Read the model definition and answer for the solid it produces. Units are mm, in the model's axes. Face numbers are marked on the shaded views. Give positions to 0.01 mm unless a question says otherwise; leave off trailing zeros. Write each loop counter-clockwise with the first axis right and the second up, starting at its lowest first coordinate (ties: lowest second). Pieces come first, ordered by that corner, then holes. Notation, with made-up numbers: (50.5, 19.5) -> (78.5, 19.5) arc R33 ccw to (78.5, 57.5) -> close; hole circle Ø5 at (71, -33). An arc over 180 degrees is marked (long way). Answer as CSV lines item,"result". Start each with the question number.
1. The part is cut by section A-A, the plane y = 0. Determine the outline of the cut face in (x, z) (3 decimals), and give its area (4 significant figures).
2. Given pin 1 (1 mm diameter, centred on x = 1.5, z = -4, fed in from +Y); pin 2 (3.5 mm diameter, centred on y = 0, z = 7.5, fed in from -X); pin 3 (1.5 mm diameter, centred on x = 1.5, z = -9.5, fed in from +Y), each flat-ended and moving along its own axis, determine where each tip first touches the part or whether it passes through.
3. For a pull along Y with two mould halves and no side action, classify the marked faces 1, 2 and 3 as pulls with the +Y half, pulls with the -Y half, needs draft (parallel to the pull), parting line crosses it, or undercut.
4. Find the intervals of material crossed by line 1 (Y direction, x = 2.55, z = 0); line 2 (Y direction, x = 2.6, z = -6.5); line 3 (Y direction, x = 1.85, z = 7.75), in increasing order.
5. The part is cut by section C-C, the plane y = 7.5. Determine the outline of the cut face in (x, z) (3 decimals), and give its area (3 significant figures).
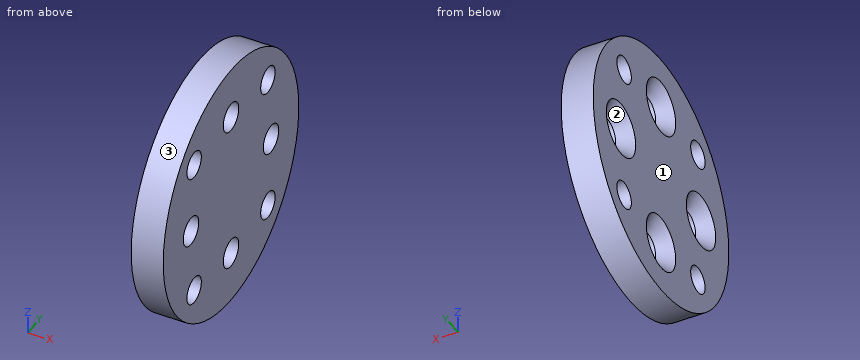
from build123d import *

# Parameters (mm, degrees)
SKETCH1_R                                         = 12.7
BOSS_EXTRUDE1_DEPTH                               = 3.175
CSK_FOR_M2_5_FLAT_HEAD_MACHINE_SCREW1_D           = 2.9
CSK_FOR_M2_5_FLAT_HEAD_MACHINE_SCREW1_CSINK_D     = 5.5
CSK_FOR_M2_5_FLAT_HEAD_MACHINE_SCREW1_CSINK_ANGLE = 90
F_6_32_TAPPED_HOLE1_D                             = 2.7051


with BuildPart() as part:
    # Sketch1 → Boss-Extrude1 (new body)
    with BuildSketch(Plane(origin=(0, 0, 0), x_dir=(0, 0, -1), z_dir=(1, 0, 0))):
        Circle(SKETCH1_R)
    extrude(amount=BOSS_EXTRUDE1_DEPTH)

    # CSK for M2.5 Flat Head Machine Screw1 (through all)
    with Locations(Plane.ZY):
        with Locations((0, 7.5), (0, -7.5), (7.5, 0), (-7.5, 0)):
            CounterSinkHole(CSK_FOR_M2_5_FLAT_HEAD_MACHINE_SCREW1_D / 2, CSK_FOR_M2_5_FLAT_HEAD_MACHINE_SCREW1_CSINK_D / 2, counter_sink_angle=CSK_FOR_M2_5_FLAT_HEAD_MACHINE_SCREW1_CSINK_ANGLE)

    # #6-32 Tapped Hole1 (through all)
    with Locations(Plane.ZY):
        with Locations((-6.914797213, 6.914797213), (-6.914797213, -6.914797213), (6.914797213, 6.914797213), (6.914797213, -6.914797213)):
            Hole(F_6_32_TAPPED_HOLE1_D / 2)


solid = part.part
Results found:
1,outline,"(0, -12.7) -> (3.175, -12.7) -> (3.175, -8.95) -> (1.3, -8.95) -> (0, -10.25) -> close; (0, -4.75) -> (1.3, -6.05) -> (3.175, -6.05) -> (3.175, 6.05) -> (1.3, 6.05) -> (0, 4.75) -> close; (0, 10.25) -> (1.3, 8.95) -> (3.175, 8.95) -> (3.175, 12.7) -> (0, 12.7) -> close"
1,area,"58.85 mm²"
2,pin 1,"stops at y = 12.21"
2,pin 2,"stops at x = 1"
2,pin 3,"stops at y = 9.2"
3,face 1,"needs draft"
3,face 2,"undercut"
3,face 3,"parting line crosses it"
4,line 1,"y = -12.7 to -8.95, -6.05 to 6.05, 8.95 to 12.7"
4,line 2,"y = -10.91 to -8.2, -5.63 to -1.05, 1.05 to 5.63, 8.2 to 10.91"
4,line 3,"y = -10.06 to -7.98, -5.85 to -1.43, 1.43 to 5.85, 7.98 to 10.06"
5,outline,"(0, -10.249) -> (3.175, -10.249) -> (3.175, -8.134) -> (0, -8.134) -> close; (0, -5.695) -> (3.175, -5.695) -> (3.175, -1.45) -> (1.3, -1.45) -> (0, -2.75) -> close; (0, 2.75) -> (1.3, 1.45) -> (3.175, 1.45) -> (3.175, 5.695) -> (0, 5.695) -> close; (0, 8.134) -> (3.175, 8.134) -> (3.175, 10.249) -> (0, 10.249) -> close"
5,area,"38.7 mm²"
